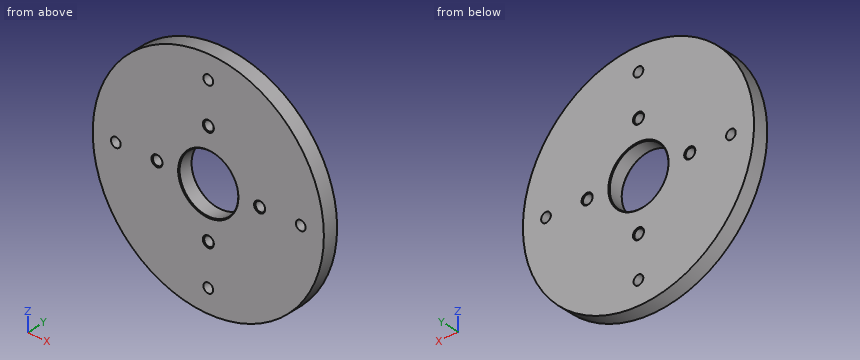
```python
from build123d import *

# Parameters (mm, degrees)
F0_R     = 75
F0_R_2   = 19.05
F1_DEPTH = 10
F2_R     = 3.1
F3_DEPTH = 10
F4_SIZE  = 0.5
F5_R     = 3.15
F6_DEPTH = 25


with BuildPart() as f1:
    # F0 (on Front) → F1 (new body)
    with BuildSketch(Plane.XZ):
        Circle(F0_R)
        Circle(F0_R_2, mode=Mode.SUBTRACT)
    extrude(amount=F1_DEPTH)

    # F2 (on face) → F3 (cut, through all)
    with BuildSketch(Plane.XZ):
        with Locations((0, 33.3047293939)):
            Circle(F2_R)
        with Locations((33.3047293939, 0)):
            Circle(F2_R)
        with Locations((0, -33.3047293939)):
            Circle(F2_R)
        with Locations((-33.3047293939, 0)):
            Circle(F2_R)
    extrude(amount=F3_DEPTH, mode=Mode.SUBTRACT)

    # F4
    f4_edges = [f1.edges().sort_by_distance(p)[0] for p in [
        (-36.404729, -10, 0),
        (-3.1, -10, 33.304729),
        (30.204729, -10, 0),
        (-3.1, -10, -33.304729),
        (-3.1, 0, -33.304729),
        (-36.404729, 0, 0),
        (-3.1, 0, 33.304729),
        (30.204729, 0, 0),
        (-19.05, 0, 0),
        (-19.05, -10, 0),
    ]]
    chamfer(f4_edges, length=F4_SIZE)

    # F5 (on face) → F6 (cut)
    with BuildSketch(Plane.XZ):
        with Locations((60, 0)):
            Circle(F5_R)
        with Locations((0, 60)):
            Circle(F5_R)
        with Locations((-60, 0)):
            Circle(F5_R)
        with Locations((0, -60)):
            Circle(F5_R)
    extrude(amount=F6_DEPTH, mode=Mode.SUBTRACT)


solid = f1.part
```
Model file for the job. Use its own axes, mm. Give positions to 0.01 mm unless a question says otherwise; leave off trailing zeros. Write each loop counter-clockwise with the first axis right and the second up, starting at its lowest first coordinate (ties: lowest second). Pieces come first, ordered by that corner, then holes. Notation, with made-up numbers: (-17, 48) -> (13, 48) arc R26 cw to (13, 83) -> close; hole circle Ø9 at (-12.5, 68.5). An arc over 180 degrees is marked (long way). Use CSV: the item, a comma, the result in double quotes. Start each with the question number.
1) Pin check, flat tips, straight feed: P1, Ø1.5, axis at x = -1.5, y = -5.5, coming from the -Z side; P2, Ø5, axis at y = -7, z = 47.5, coming from the -X side; P3, Ø1, axis at y = -5.5, z = 38.5, coming from the +X side. Stop position of each tip, or through.
2) Cut at B-B on z = 60. List the corners of the cut face in (x, y), plus the area to 3 significant figures.
3) Drill centre lines: L1, parallel to Z at x = 0, y = -3.5; L2, parallel to X at y = -3.75, z = 61; L3, parallel to X at y = -1.5, z = 4. Where is each one in solid material? Low to high.
4) Cut at A-A on x = -60. List the corners of the cut face in (y, z).
5) Cut at C-C on z = 0. Count the separate pieces of the cut face and the enclosed holes in it, plus the area to 4 significant figures.
Final values:
1,P1,"stops at z = -75"
1,P2,"stops at x = -60"
1,P3,"stops at x = 64.66"
2,outline,"(-45, -10) -> (-3.15, -10) -> (-3.15, 0) -> (-45, 0) -> close; (3.15, -10) -> (45, -10) -> (45, 0) -> (3.15, 0) -> close"
2,area,"837 mm2"
3,L1,"z = -75 to -63.15, -56.85 to -36.4, -30.2 to -19.05, 19.05 to 30.2, 36.4 to 56.85, 63.15 to 75"
3,L2,"x = -43.63 to -2.99, 2.99 to 43.63"
3,L3,"x = -74.89 to -18.63, 18.63 to 74.89"
4,outline,"(-10, -45) -> (0, -45) -> (0, -3.15) -> (-10, -3.15) -> close; (-10, 3.15) -> (0, 3.15) -> (0, 45) -> (-10, 45) -> close"
5,separate pieces,"6"
5,enclosed holes,"0"
5,area,"867.5 mm2"
